The model under review builds one solid part; all positions refer to its coordinate system, in mm. Round coordinates to 2 decimals unless told otherwise and drop trailing zeros. Answer as a JSON object with one key per item and string values. Group by question number.
1) Insertion check: pin 1 Ø6.5 at (x, y) = (-55.98, -89.66) entering from +Z; pin 2 Ø0.8 at (y, z) = (-10.5, 1) entering from +X. Each pin has a flat end and moves straight along its axis. Give the tip position at first contact, or say it passes through.
2) Consider section A-A, the plane z = 0.7. Count the separate pieces of the cut face and the enclosed holes in it, then the cut area to 3 significant figures.
3) To check wall thickness, follow line 1 (X direction, y = -31.5, z = 0.3); line 2 (Y direction, x = 18.5, z = 1.25); line 3 (Y direction, x = -21.5, z = 1.05). State the ranges of each line that lie inside material, in increasing order.
```python
from build123d import *

# Parameters (mm, degrees)
EXTRUDE_1_DEPTH     = 1.5
HOLE_WIZARD_M4_1_D  = 4.2
HOLE_WIZARD_M8_1_D  = 8.25
SKETCH_8_R          = 3.5
CUT_EXTRUDE_1_DEPTH = 144.323608762
SKETCH_9_R          = 3.5
CUT_EXTRUDE_2_DEPTH = 144.323608762
CUT_EXTRUDE_3_DEPTH = 144.323608762


with BuildPart() as part:
    # 草圖1 → 填料-伸長1 (new body)
    with BuildSketch(Plane.XY):
        with BuildLine():
            Line((9.519190028, -18.946187519), (9.519190028, -5.659090909))
            ThreePointArc((9.519190028, -5.659090909), (9.226296809, -4.951984128), (8.519190028, -4.659090909))
            Line((8.519190028, -4.659090909), (-70.48081017, -4.659090909))
            ThreePointArc((-70.48081017, -4.659090909), (-71.187916951, -4.951984128), (-71.48081017, -5.659090909))
            Line((-71.48081017, -5.659090909), (-71.48081017, -18.946187519))
            ThreePointArc((-71.48081017, -18.946187519), (-73.531062702, -23.895934988), (-78.48081017, -25.946187519))
            Line((-78.48081017, -25.946187519), (-84.980810071, -25.946187519))
            ThreePointArc((-84.980810071, -25.946187519), (-85.687916853, -26.239080738), (-85.980810071, -26.946187519))
            Line((-85.980810071, -26.946187519), (-85.980810071, -92.341911374))
            ThreePointArc((-85.980810071, -92.341911374), (-85.688840793, -93.048093006), (-84.983425077, -93.341907955))
            Line((-84.983425077, -93.341907955), (-78.583599692, -93.358643592))
            ThreePointArc((-78.583599692, -93.358643592), (-73.586751521, -95.475153852), (-71.603919064, -100.526538095))
            Line((-71.603919064, -100.526538095), (-71.918462387, -113.635102561))
            ThreePointArc((-71.918462387, -113.635102561), (-71.634287831, -114.357665047), (-70.918750149, -114.659090909))
            Line((-70.918750149, -114.659090909), (8.519190028, -114.659090909))
            ThreePointArc((8.519190028, -114.659090909), (9.226296809, -114.36619769), (9.519190028, -113.659090909))
            Line((9.519190028, -113.659090909), (9.519190028, -100.371994299))
            ThreePointArc((9.519190028, -100.371994299), (11.569442559, -95.422246831), (16.519190028, -93.371994299))
            Line((16.519190028, -93.371994299), (23.019189929, -93.371994299))
            ThreePointArc((23.019189929, -93.371994299), (23.72629671, -93.07910108), (24.019189929, -92.371994299))
            Line((24.019189929, -92.371994299), (24.019189929, -26.946187519))
            ThreePointArc((24.019189929, -26.946187519), (23.72629671, -26.239080738), (23.019189929, -25.946187519))
            Line((23.019189929, -25.946187519), (16.519190028, -25.946187519))
            ThreePointArc((16.519190028, -25.946187519), (11.569442559, -23.895934988), (9.519190028, -18.946187519))
        make_face()
    extrude(amount=EXTRUDE_1_DEPTH)

    # M4 螺旋的螺孔鑽1 (through all)
    with Locations(Plane(origin=(0, 0, 0), x_dir=(-1, 0, 0), z_dir=(0, 0, -1))):
        with Locations((79.980810071, -87.644049447), (-18.019189929, -87.644049447), (-18.019189929, -31.644049447), (79.980810071, -31.644049447)):
            Hole(HOLE_WIZARD_M4_1_D / 2)

    # M8 螺旋的螺孔鑽1 (through all)
    with Locations(Plane.XY.offset(1.5)):
        with Locations((-55.980810071, -89.659090909), (-25.980810071, -89.659090909)):
            Hole(HOLE_WIZARD_M8_1_D / 2)

    # 草圖8 → 除料-伸長1 (cut, through all)
    with BuildSketch(Plane.XY.offset(1.5)):
        with Locations((4.019190028, -101.159090909)):
            Circle(SKETCH_8_R)
    extrude(amount=-CUT_EXTRUDE_1_DEPTH, mode=Mode.SUBTRACT)

    # 草圖9 → 除料-伸長2 (cut, through all)
    with BuildSketch(Plane.XY.offset(1.5)):
        with Locations((-0.480809972, -13.659090909)):
            Circle(SKETCH_9_R)
        with Locations((-20.480809972, -13.659090909)):
            Circle(SKETCH_9_R)
    extrude(amount=-CUT_EXTRUDE_2_DEPTH, mode=Mode.SUBTRACT)

    # 草圖10 → 除料-伸長3 (cut, through all)
    with BuildSketch(Plane.XY.offset(1.5)):
        with BuildLine():
            Line((-50.230810071, -91.159090909), (-50.230810071, -88.159090909))
            ThreePointArc((-50.230810071, -88.159090909), (-49.480810071, -87.409090909), (-48.730810071, -88.159090909))
            Line((-48.730810071, -88.159090909), (-48.730810071, -91.159090909))
            ThreePointArc((-48.730810071, -91.159090909), (-49.480810071, -91.909090909), (-50.230810071, -91.159090909))
        make_face()
        with BuildLine():
            Line((-20.230810071, -91.159090909), (-20.230810071, -88.159090909))
            ThreePointArc((-20.230810071, -88.159090909), (-19.480810071, -87.409090909), (-18.730810071, -88.159090909))
            Line((-18.730810071, -88.159090909), (-18.730810071, -91.159090909))
            ThreePointArc((-18.730810071, -91.159090909), (-19.480810071, -91.909090909), (-20.230810071, -91.159090909))
        make_face()
    extrude(amount=-CUT_EXTRUDE_3_DEPTH, mode=Mode.SUBTRACT)


solid = part.part
```
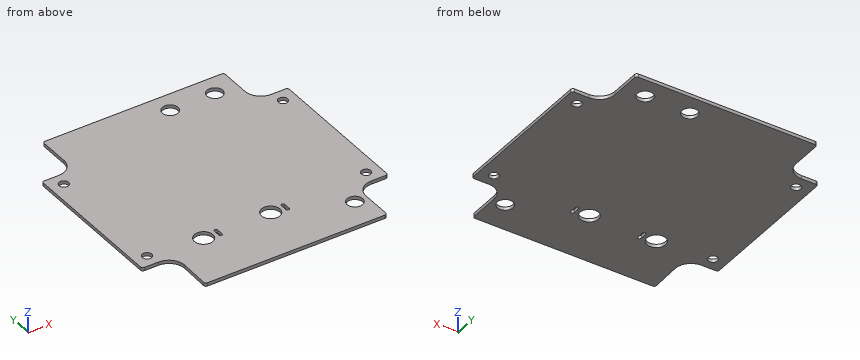
Results list:
{
 "1": {"pin 1": "through", "pin 2": "x = 9.52"},
 "2": {"separate pieces": "1", "enclosed holes": "11", "area": "10,600 mm^2"},
 "3": {"line 1": "-85.98 to -82.08, -77.89 to 15.92, 20.11 to 24.02", "line 2": "-93.37 to -89.69, -85.6 to -33.69, -29.6 to -25.95", "line 3": "-114.66 to -17.01, -10.31 to -4.66"}
}
